```python
from build123d import *

# Parameters (mm, degrees)
F1_R     = 9
F2_DEPTH = 10


with BuildPart() as f2:
    # F1 (on offset) → F2 (new body)
    with BuildSketch(Plane.XZ.offset(1)):
        Polygon((20, -70), (20, 20), (-20, 20), (-20, -59.039845), (-9.039845, -70), align=None)
        Circle(F1_R, mode=Mode.SUBTRACT)
    extrude(amount=F2_DEPTH)


solid = f2.part
```
Part model, mm, in its own coordinate system. Coordinates: 2 decimals unless noted, no trailing zeros. Loops run counter-clockwise (first coordinate to the right, second up) from the corner with the lowest first, then second, coordinate; pieces in that order, holes last. Notation, with made-up numbers: (29.25, -3) - (78.25, -3) arc R24 cw to (78.25, 11) - close; hole circle Ø11 at (37.25, -12.75). An arc over 180 degrees is marked (long way). Write item = value, one per line. Start each with the question number.
Item 1: Cut at B-B, the plane y = -6. Give the cut face in (x, z), and give its area (3 significant figures).
Item 2: Cut at C-C, the plane x = 0. Give the cut face in (y, z), and give its area (3 significant figures).
Item 3: Wall check: L1, parallel to Z at x = 0, y = -3.5; L2, parallel to X at y = -4, z = 7; L3, parallel to X at y = -2.25, z = 6. Give the ranges that are in metal, low to high. Write a range as from..to.
Item 4: Mould opens along X. For faces 1 (the flat face through (20, -6, -26)), 2 (the cylindrical face through (-1.172, -5.93, 8.923)), 3 (the flat face through (5, -6, -70)) say: released by +X, released by -X, zero draft, split by the parting line, or undercut.
Item 5: Cut at A-A, the plane z = 0. Give the cut face in (x, y), and give its area (3 significant figures).
The answers:
q1.outline = (-20, -59.04) - (-9.04, -70) - (20, -70) - (20, 20) - (-20, 20) - close; hole circle Ø18 at (0, 0)
q1.area = 3,290 mm2
q2.outline = (-11, -70) - (-1, -70) - (-1, -9) - (-11, -9) - close; (-11, 9) - (-1, 9) - (-1, 20) - (-11, 20) - close
q2.area = 720 mm2
q3.L1 = -70..-9, 9..20
q3.L2 = -20..-5.66, 5.66..20
q3.L3 = -20..-6.71, 6.71..20
q4.face_1 = released by +X
q4.face_2 = undercut
q4.face_3 = zero draft
q5.outline = (-20, -11) - (-9, -11) - (-9, -1) - (-20, -1) - close; (9, -11) - (20, -11) - (20, -1) - (9, -1) - close
q5.area = 220 mm2
